Design review of the part built by this model. Coordinates are the model's own, in mm. Face numbers are marked on the shaded views. A direction names the side the tool comes from. Give positions to 0.01 mm unless a question says otherwise; leave off trailing zeros. Write each loop counter-clockwise with the first axis right and the second up, starting at its lowest first coordinate (ties: lowest second). Pieces come first, ordered by that corner, then holes. Notation, with made-up numbers: (42.25, 8) -> (79.25, 8) arc R12 ccw to (79.25, 21) -> close; hole circle Ø8 at (32, -2.75). An arc over 180 degrees is marked (long way). Answer as a JSON object with one key per item and string values.
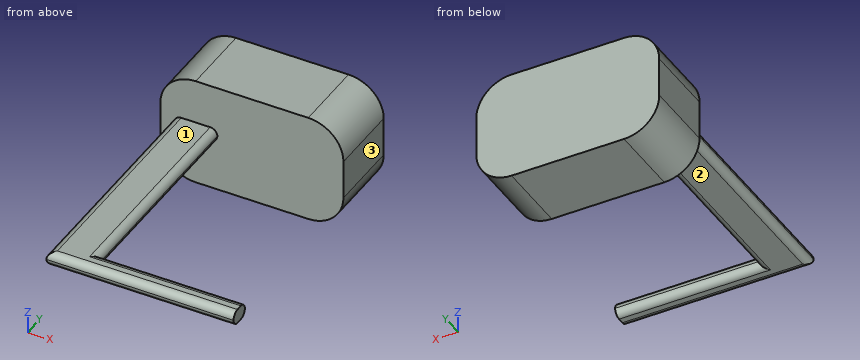
```python
from build123d import *

# Parameters (mm, degrees)
F0_W     = 127
F0_H     = 76.2
F1_DEPTH = 50.8
F2_R     = 24.4421069165
F4_W     = 30
F4_H     = 10
F5_DEPTH = 211.9498550892
F6_W     = 14.2212212086
F6_H     = 10
F7_DEPTH = 100
F8_R     = 4.99999


# Not quite as in the source:
# - a fillet or chamfer is up to 0.001 mm smaller than in the source, because OpenCascade refuses the exact size


with BuildPart() as f1:
    # F0 (on Front) → F1 (new body)
    with BuildSketch(Plane.XZ):
        with Locations((21.6533541679, 32.7783897177)):
            Rectangle(F0_W, F0_H)
    extrude(amount=F1_DEPTH)

    # F2
    f2_edges = [f1.edges().sort_by_distance(p)[0] for p in [
        (-41.846646, -25.4, 70.87839),
        (-41.846646, -25.4, -5.32161),
        (85.153354, -25.4, -5.32161),
        (85.153354, -25.4, 70.87839),
    ]]
    fillet(f2_edges, radius=F2_R)

    # F4 (on face) → F5 (join)
    with BuildSketch(Plane(origin=(0, 0, 0), x_dir=(-1, 0, 0), z_dir=(0, 1, 0))):
        with Locations((17.3587081618, 34.757822752)):
            Rectangle(F4_W, F4_H)
    extrude(amount=-F5_DEPTH)

    # F6 (on face) → F7 (join)
    with BuildSketch(Plane.YZ.offset(-2.3587081618)):
        with Locations((-204.8392444849, 34.757822752)):
            Rectangle(F6_W, F6_H)
    extrude(amount=F7_DEPTH)

    # F8 (radius 5 in the source; OpenCascade refuses exactly that, so slightly less here)
    f8_edges = [f1.edges().sort_by_distance(p)[0] for p in [
        (-32.358708, -131.374928, 39.757823),
        (-32.358708, -131.374928, 29.757823),
        (32.641292, -211.949855, 29.757823),
        (-2.358708, -124.264317, 29.757823),
        (-2.358708, -124.264317, 39.757823),
        (47.641292, -197.728634, 39.757823),
        (32.641292, -211.949855, 39.757823),
        (47.641292, -197.728634, 29.757823),
    ]]
    fillet(f8_edges, radius=F8_R)


solid = f1.part
```
(1) We need section C-C, the plane z = 32. State the section outline as (x, y) points.
Here are the results:
{"outline": "(-41.85, -50.8) -> (-31.53, -50.8) -> (-31.53, -211.12) -> (97.64, -211.12) -> (97.64, -198.56) -> (-3.19, -198.56) -> (-3.19, -50.8) -> (85.15, -50.8) -> (85.15, 0) -> (-41.85, 0) -> close"}
(2) Clearance check with flat-ended pins moving along their axes: pin 1 (12 mm diameter, centred on x = 65.5, z = 29, fed in from -Y); pin 2 (1.5 mm diameter, centred on y = -26, z = 56.5, fed in from -X); pin 3 (1.5 mm diameter, centred on x = 52.5, z = 7.5, fed in from -Y). State where each tip first meets the part, or that it passes through.
Here are the results:
{"pin 1": "stops at y = -211.95", "pin 2": "stops at x = -40", "pin 3": "stops at y = -50.8"}
(3) For line 1 along Z through (x, y) = (-12, -90.5); line 2 along Y through (x, z) = (79, 44); line 3 along X through (y, z) = (-41.5, 23), list the stretches that pass through material, from the lowest coordinate up.
Here are the results:
{"line 1": "z = 29.76 to 39.76", "line 2": "y = -50.8 to 0", "line 3": "x = -41.85 to 85.15"}
(4) For the marked faces 1, 2 and 3, list the 3-axis set-ups (+Z, -Z, +X, -X, +Y, -Y) from which the entire face can be reached by the end or side of a thin tool; tool diameter is ignored.
Here are the results:
{"face 1": "+Z, +X, -X, -Y", "face 2": "-Z, +X, -X, -Y", "face 3": "+Z, -Z, +X, +Y"}
(5) We need section D-D, the plane y = -34. State the section outline as (x, z) points.
Here are the results:
{"outline": "(-41.85, 19.12) arc R24.44 ccw to (-17.4, -5.32) -> (60.71, -5.32) arc R24.44 ccw to (85.15, 19.12) -> (85.15, 46.44) arc R24.44 ccw to (60.71, 70.88) -> (-17.4, 70.88) arc R24.44 ccw to (-41.85, 46.44) -> close"}
